Autodesk Inventor part; units mm, degrees
ref_plane "작업 평면1" through (0, 0, 8.3) normal (0, 0, 1) x (1, 0, 0)
ref_plane "YZ Plane" through (0, 0, 0) normal (1, 0, 0) x (0, 1, 0)
ref_plane "XZ Plane" through (0, 0, 0) normal (0, 1, 0) x (-1, 0, 0)
sketch "스케치1" plane through (0, 0, 0) normal (1, 0, 0) x (0, 1, 0)
  circle A0 centre (0, 0) radius 5.3
  circle A1 centre (0, 0) radius 5
  line L0 (4, 3) -> (-4, 3)
  circle A2 centre (0, 0) radius 8.3
  line L1 (4, 3) -> (11.6093, 3)
  line L2 (-4, 3) -> (-10.334, 3)
  line L3 (11.6093, -38.4) -> (-10.334, -38.4) construction
  circle A3 centre (0, -76.8) radius 5.3
  circle A4 centre (0, -76.8) radius 5
  line L4 (4, -79.8) -> (-4, -79.8)
  circle A5 centre (0, -76.8) radius 8.3
  line L5 (4, -79.8) -> (11.6093, -79.8)
  line L6 (-4, -79.8) -> (-10.334, -79.8)
  line L7 (-8.3, 0) -> (-8.3, -76.8)
  line L8 (-5.3, 0) -> (-5.3, -76.8)
  line L9 (0, -8.3) -> (-5.3, -8.3)
  line L10 (0, -68.5) -> (-5.3, -68.5)
  point P0 (0, 3)
  point P1 (0, -79.8)
  point P2 (-4.3692, -79.8)
  point P3 (4.3692, -79.8)
  point P4 (7.7389, 3)
  point P5 (4.3692, 3)
  point P6 (-4.3692, 3)
  point P7 (-7.7389, 3)
  point P8 (-7.7389, -79.8)
  point P9 (7.7389, -79.8)
  dimension "d0" = 10.6
  dimension "d1" = 3
  dimension "d2" = 10
  dimension "d3" = 16.6
  dimension "d4" = 38.4
extrude "돌출1" add sketch "스케치1" along normal blind 20 contours L8 A2 L2 A0 | A0 L1 A2 L8 | L8 A5 L7 A2 | A2 L9 L8 | A5 L8 A3 L6 | L10 A5 L8 | A5 L5 A3 L8
ref_plane "작업 평면1" through (0, 0, 8.3) normal (0, 0, 1) x (1, 0, 0)
sketch "스케치2" plane through (0, 0, 8.3) normal (0, 0, 1) x (1, 0, 0)
  line L0 (0, 4.3692) -> (20, 4.3692)
  line L1 (0, 0) -> (0, 7.7389)
  line L2 (0, -8.3) -> (20, -8.3)
  line L3 (20, 0) -> (20, 7.7389)
  line L4 (0, 0) -> (20, 0)
  line L5 (0, 8.3) -> (20, 8.3)
  circle A0 centre (10, 0) radius 1.25
  line L6 (0, 7.7389) -> (20, 7.7389)
  line L7 (0, -7.7389) -> (0, -8.3)
  line L8 (20, -7.7389) -> (20, -8.3)
  line L9 (0, -7.7389) -> (20, -7.7389)
  point P0 (0, 0)
  dimension "d7" = 2.5
extrude "돌출2" cut sketch "스케치2" along normal through all both and the other way through all contours A0 L4 | L4 A0
sketch "스케치3" plane through (0, -8.3, -76.8) normal (0, -1, 0) x (1, 0, 0)
  line L0 (0, 76.8) -> (0, 0)
  line L1 (0, 0) -> (20, 0)
  line L2 (20, 76.8) -> (20, 0)
  line L3 (0, 76.8) -> (20, 76.8)
  line L4 (0, 0) -> (0, -3)
  line L5 (0, -3) -> (20, -3)
  line L6 (20, 0) -> (20, -3)
  line L7 (0, 0) -> (20, 0)
  line L8 (0, 79.8) -> (0, 76.8)
  line L9 (0, 76.8) -> (20, 76.8)
  line L10 (20, 79.8) -> (20, 76.8)
  line L11 (0, 79.8) -> (20, 79.8)
  line L12 (20, 38.4) -> (0, 38.4) construction
  line L13 (0, 79.8) -> (20, 79.8)
  line L14 (10, 79.8) -> (10, -3) construction
  circle A0 centre (10, 19.2) radius 2.5
  line L15 (6, 12.3) -> (14, 12.3)
  line L16 (14, 12.3) -> (14, 4.3)
  line L17 (14, 4.3) -> (6, 4.3)
  line L18 (6, 4.3) -> (6, 12.3)
  line L19 (0, 8.3) -> (20, 8.3)
  line L20 (6, 12.3) -> (14, 4.3) construction
  line L21 (14, 12.3) -> (6, 4.3) construction
  circle A1 centre (10, 57.6) radius 2.5
  line L22 (6, 64.5) -> (14, 64.5)
  line L23 (14, 64.5) -> (14, 72.5)
  line L24 (14, 72.5) -> (6, 72.5)
  line L25 (6, 72.5) -> (6, 64.5)
  line L26 (0, 68.5) -> (20, 68.5)
  line L27 (6, 64.5) -> (14, 72.5) construction
  line L28 (14, 64.5) -> (6, 72.5) construction
  point P0 (10, 8.3)
  point P1 (10, 68.5)
  dimension "d10" = 38.4
  dimension "d11" = 10
  dimension "d12" = 5
  dimension "d13" = 19.2
  dimension "d14" = 8
  dimension "d15" = 8
extrude "돌출3" cut sketch "스케치3" against normal blind 20 contours A0 | A1
extrude "돌출4" add sketch "스케치3" along normal blind 2 contours L26 L23 L22 L25 | L25 L24 L23 L26 | L19 L16 L17 L18 | L18 L15 L16 L19
properties part number "pipe_holder_typeA"
Geometry check sheet. Reference: the model listing, model coordinates, mm. A direction names the side the tool comes from. Coordinates: 2 decimals unless noted, no trailing zeros. Write each loop counter-clockwise with the first axis right and the second up, starting at its lowest first coordinate (ties: lowest second). Pieces come first, ordered by that corner, then holes. Notation, with made-up numbers: M 79,-31 L 105,-31 A11 ccw 105,-23 Z; hole C 54,-3 d1. An arc over 180 degrees is marked long. Use one line per item in the form item = value. Start each with the question number.
1) Section check A-A on z = -19.2. Enter the section's corners in (x, y).
2) Thickness scan on probe 1 along Z at (x, y) = (10, -7.2); probe 2 along Z at (x, y) = (5.5, 0); probe 3 along Y at (x, z) = (6, 0). Record the ranges inside material, lowest first. Write a range as from..to.
3) Set-up check for faces 1 (the flat face through (10, -9, -12.3)), 2 (the flat face through (10, -9, -72.5)), 3 (the flat face through (10, -9, -4.3)), 4 (the cylindrical face through (11.15, -6.82, -21.42)): record each of +Z, -Z, +X, -X, +Y, -Y from which the full face is reachable in a straight line by a thin tool's end or side.
4) Section check C-C on x = 16.5. Enter the section's corners in (y, z), and give its area (3 significant figures).
5) Section check D-D on z = -65.5. Enter the section's corners in (x, y).
6) Go/stop test with flat-tipped pins: pin 1 Ø6 at (x, z) = (6.5, -21.5) entering from -Y; pin 2 Ø10 at (x, z) = (11, -58) entering from +Y; pin 3 Ø0.6 at (y, z) = (-9.5, -68) entering from +X. Record where each tip stops, or that it passes through.
7) Section check B-B on y = -2.25. Enter the section's corners in (x, z).
8) Release check for a two-part mould opening along X. For faces 5 (the cylindrical face through (8.75, 0.05, -70.05)), 6 (the flat face through (20, -6, -38)), 7 (the flat face through (10, -10.3, -68)) record: pulls with the +X half, pulls with the -X half, needs draft (parallel to the pull), parting line crosses it, or undercut.
Responses:
q1.outline = M 0,-8.3 L 7.5,-8.3 L 7.5,-5.3 L 0,-5.3 Z; M 12.5,-8.3 L 20,-8.3 L 20,-5.3 L 12.5,-5.3 Z
q2.probe_1 = -79.8..-60.1, -55.1..-21.7, -16.7..3
q2.probe_2 = -71.5..-68.5, -8.3..-5.3
q2.probe_3 = -8.3..-5.3, 5.3..8.3
q3.face_1 = +X, -X, -Y
q3.face_2 = -Z, +X, -X, -Y
q3.face_3 = +Z, +X, -X, -Y
q3.face_4 = +Y, -Y
q4.outline = M -8.3,-76.8 A8.3 ccw -7.74,-79.8 L -4.37,-79.8 A5.3 cw long 4.37,-79.8 L 7.74,-79.8 A8.3 ccw 0,-68.5 L -5.3,-68.5 L -5.3,-8.3 L 0,-8.3 A8.3 ccw 7.74,3 L 4.37,3 A5.3 cw long -4.37,3 L -7.74,3 A8.3 ccw -8.3,0 Z
q4.area = 376 mm2
q5.outline = M 0,-8.3 L 6,-8.3 L 6,-10.3 L 14,-10.3 L 14,-8.3 L 20,-8.3 L 20,-5.3 L 0,-5.3 Z
q6.pin_1 = -8.3
q6.pin_2 = -5.3
q6.pin_3 = 14
q7.outline = M 0,-72 L 20,-72 L 20,-68.5 L 0,-68.5 Z; M 0,-8.3 L 20,-8.3 L 20,-4.8 L 0,-4.8 Z
q8.face_5 = undercut
q8.face_6 = pulls with the +X half
q8.face_7 = needs draft
